```python
from build123d import *

# Parameters (mm, degrees)
SKETCH2_R           = 116.84
BOSS_EXTRUDE1_DEPTH = 1.5875
SKETCH3_W           = 232.210592103
SKETCH3_H           = 398.954583541
CUT_EXTRUDE1_DEPTH  = 133.08
SKETCH4_W           = 3.3782
SKETCH4_H           = 10.16
CUT_EXTRUDE2_DEPTH  = 4.175


with BuildPart() as part:
    # Sketch2 → Boss-Extrude1 (new body, symmetric)
    with BuildSketch(Plane.XY):
        with BuildLine():
            ThreePointArc((-1.651, 128.513680847), (-113.443755652, 64.087482344), (-116.974071472, -64.89271823))
            ThreePointArc((-116.974071472, -64.89271823), (-116.588202689, -65.623039511), (-116.197774242, -66.350933404))
            ThreePointArc((-116.197774242, -66.350933404), (-115.802941233, -67.076116512), (-115.403582459, -67.798817153))
            ThreePointArc((-115.403582459, -67.798817153), (0, -135.636), (115.403582459, -67.798817153))
            ThreePointArc((115.403582459, -67.798817153), (115.802941375, -67.076116254), (116.197774523, -66.350932884))
            ThreePointArc((116.197774523, -66.350932884), (116.588202828, -65.62303925), (116.974071472, -64.89271823))
            ThreePointArc((116.974071472, -64.89271823), (113.443755652, 64.087482344), (1.651, 128.513680847))
            ThreePointArc((1.651, 128.513680847), (0.825516124, 128.521420187), (0, 128.524))
            ThreePointArc((0, 128.524), (-0.825516124, 128.521420187), (-1.651, 128.513680847))
        make_face()
        with Locations((0, -3.556)):
            Circle(SKETCH2_R, mode=Mode.SUBTRACT)
    extrude(amount=BOSS_EXTRUDE1_DEPTH, both=True)

    # Sketch3 → Cut-Extrude1 (cut, through all)
    with BuildSketch(Plane(origin=(0, 0, 0), x_dir=(0, 0, -1), z_dir=(1, 0, 0))):
        with Locations((6.714523145, -6.913261573)):
            Rectangle(SKETCH3_W, SKETCH3_H)
    extrude(amount=CUT_EXTRUDE1_DEPTH, mode=Mode.SUBTRACT)

    # Sketch4 → Cut-Extrude2 (cut, through all)
    with BuildSketch(Plane.XY.offset(1.5875)):
        with Locations((-1.6891, 124.714)):
            Rectangle(SKETCH4_W, SKETCH4_H)
        Polygon((-105.620566898, 59.765541567), (-103.931466898, 62.691148586), (-112.730285, 67.771148586), (-114.419385, 64.845541567), align=None)
        with Locations((-1.6891, -131.826)):
            Rectangle(SKETCH4_W, SKETCH4_H)
        Polygon((-107.648347053, -63.365323312), (-109.337447053, -60.439716293), (-118.136265155, -65.519716293), (-116.447165155, -68.445323312), align=None)
    extrude(amount=-CUT_EXTRUDE2_DEPTH, mode=Mode.SUBTRACT)


solid = part.part
```
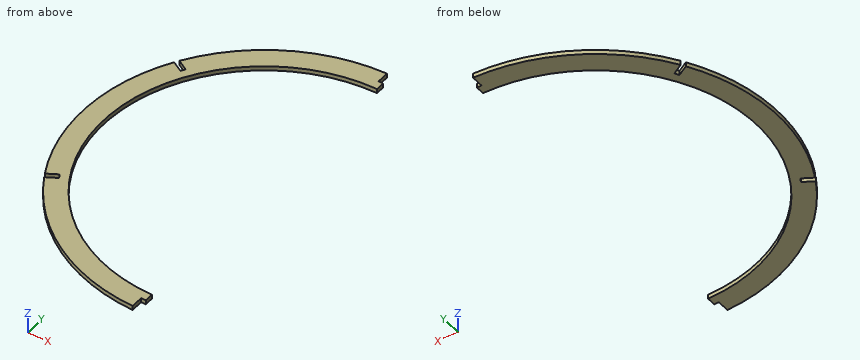
The model under review builds one solid part; all positions refer to its coordinate system, in mm. Round coordinates to 2 decimals unless told otherwise and drop trailing zeros. Write each loop counter-clockwise with the first axis right and the second up, starting at its lowest first coordinate (ties: lowest second). Pieces come first, ordered by that corner, then holes. Notation, with made-up numbers: (5.25, 73) - (48.25, 73) arc R25 ccw to (48.25, 110) - close; hole circle Ø7 at (70, -12). An arc over 180 degrees is marked (long way). Answer as CSV lines item,"result". Start each with the question number.
(1) We need section A-A on x = -83. State the section outline as (y, z) points.
(2) For pin 1 Ø1 at (x, z) = (-2, 0) entering from +Y; pin 2 Ø1.6 at (y, z) = (-131.5, 0.5) entering from +X; pin 3 Ø1.5 at (x, z) = (-53.5, 0.5) entering from +Y, all flat-tipped, find the tip position at first contact; note any pin that passes through.
(3) We need section C-C on x = -7.5. State the section outline as (y, z) points.
(4) We need section D-D on y = -16. State the section outline as (x, z) points, plus the area to 3 significant figures.
(5) To check wall thickness, follow line 1 (Y direction, x = -27, z = -1.4); line 2 (Y direction, x = -48.5, z = -1.1); line 3 (X direction, y = -121, z = -0.45). State the ranges of each line that lie inside material, in increasing order.
(6) We need section B-B on z = -0.85. State the section outline as (x, y) points, plus the area to 3 significant figures.
Worked answers:
1,outline,"(-106.3, -1.59) - (-85.79, -1.59) - (-85.79, 1.59) - (-106.3, 1.59) - close; (78.68, -1.59) - (99.19, -1.59) - (99.19, 1.59) - (78.68, 1.59) - close"
2,pin 1,"y = 119.63"
2,pin 2,"x = -3.38"
2,pin 3,"y = 117.53"
3,outline,"(-135.42, -1.59) - (-120.16, -1.59) - (-120.16, 1.59) - (-135.42, 1.59) - close; (113.04, -1.59) - (128.31, -1.59) - (128.31, 1.59) - (113.04, 1.59) - close"
4,outline,"(-131.49, -1.59) - (-116.18, -1.59) - (-116.18, 1.59) - (-131.49, 1.59) - close"
4,area,"48.6 mm²"
5,line 1,"-132.85 to -117.23, 110.12 to 125.73"
5,line 2,"-126.41 to -109.85, 102.74 to 119.3"
5,line 3,"-60.43 to 0"
6,outline,"(-116.99, -64.86) - (-109.34, -60.44) - (-107.65, -63.37) - (-115.39, -67.83) arc R132.08 ccw to (-3.38, -135.59) - (-3.38, -126.75) - (0, -126.75) - (0, -120.4) arc R116.84 cw to (0, 113.28) - (0, 119.63) - (-3.38, 119.63) - (-3.38, 128.48) arc R132.08 ccw to (-111.59, 67.11) - (-103.93, 62.69) - (-105.62, 59.77) - (-113.36, 64.23) arc R132.08 ccw to start"
6,area,"5,840 mm²"
